```python
from build123d import *

# Parameters (mm, degrees)
SKETCH_1_R          = 50
EXTRUDE_1_DEPTH     = 15
SHELL_1_T           = -3
EXTRUDE_2_DEPTH     = 20
SKETCH_3_R          = 13
CUT_EXTRUDE_1_DEPTH = 79.89866919
SKETCH_4_R          = 16
SKETCH_4_R_2        = 13
EXTRUDE_3_DEPTH     = 12
SHELL_START         = 15
SHELL_5_DEPTH       = 20


# Read off the part's stored shape, not the designer's step: 薄殼5
with BuildPart() as part:
    # 草圖1 → 填料-伸長1 (new body)
    with BuildSketch(Plane.XY):
        Circle(SKETCH_1_R)
    extrude(amount=EXTRUDE_1_DEPTH)

    # 薄殼1
    shell_1_openings = [part.faces().sort_by_distance(p)[0] for p in [
        (0, 0, 0),
    ]]
    offset(amount=SHELL_1_T, openings=shell_1_openings, kind=Kind.INTERSECTION)

    # 草圖2 → 填料-伸長2 (add)
    with BuildSketch(Plane.XY.offset(15)):
        with BuildLine():
            Line((-15.588457268, 33), (-36.373066959, -3))
            ThreePointArc((-36.373066959, -3), (-36.373066959, -21), (-20.784609691, -30))
            Line((-20.784609691, -30), (20.784609691, -30))
            ThreePointArc((20.784609691, -30), (36.373066959, -21), (36.373066959, -3))
            Line((36.373066959, -3), (15.588457268, 33))
            ThreePointArc((15.588457268, 33), (0, 42), (-15.588457268, 33))
        make_face()
    extrude(amount=EXTRUDE_2_DEPTH)

    # 草圖3 → 除料-伸長1 (cut, through all)
    with BuildSketch(Plane.XY.offset(35)):
        with Locations((0, 24)):
            Circle(SKETCH_3_R)
        with Locations((-20.784609691, -12)):
            Circle(SKETCH_3_R)
        with Locations((20.784609691, -12)):
            Circle(SKETCH_3_R)
    extrude(amount=-CUT_EXTRUDE_1_DEPTH, mode=Mode.SUBTRACT)

    # 草圖4 → 填料-伸長3 (add)
    # profile 1 of 3: a face of its own
    with BuildSketch(Plane(origin=(0, 0, 12), x_dir=(-1, 0, 0), z_dir=(0, 0, -1))):
        with Locations(Location((0, 24, 0), (0, 0, 180))):
            Circle(SKETCH_4_R)
        with Locations(Location((0, 24, 0), (0, 0, 180))):
            Circle(SKETCH_4_R_2, mode=Mode.SUBTRACT)
    # profile 2 of 3: a face of its own
    with BuildSketch(Plane(origin=(0, 0, 12), x_dir=(-1, 0, 0), z_dir=(0, 0, -1))):
        with Locations(Location((20.784609691, -12, 0), (0, 0, 180))):
            Circle(SKETCH_4_R)
        with Locations(Location((20.784609691, -12, 0), (0, 0, 180))):
            Circle(SKETCH_4_R_2, mode=Mode.SUBTRACT)
    # profile 3 of 3: a face of its own
    with BuildSketch(Plane(origin=(0, 0, 12), x_dir=(-1, 0, 0), z_dir=(0, 0, -1))):
        with Locations(Location((-20.784609691, -12, 0), (0, 0, 180))):
            Circle(SKETCH_4_R)
        with Locations(Location((-20.784609691, -12, 0), (0, 0, 180))):
            Circle(SKETCH_4_R_2, mode=Mode.SUBTRACT)
    extrude(amount=EXTRUDE_3_DEPTH)

    # 薄殼5 outline → 薄殼5 (cut)
    with BuildSketch(Plane.XY.offset(SHELL_START)):
        with BuildLine():
            ThreePointArc((15.774263238, 26.67817462), (0, 8), (-15.774263238, 26.67817462))
            Line((-15.774263238, 26.67817462), (-30.991108566, 0.32182538))
            ThreePointArc((-30.991108566, 0.32182538), (-6.92820323, -4), (-15.216845328, -27))
            Line((-15.216845328, -27), (15.216845328, -27))
            ThreePointArc((15.216845328, -27), (6.92820323, -4), (30.991108566, 0.32182538))
            Line((30.991108566, 0.32182538), (15.774263238, 26.67817462))
        make_face()
    extrude(amount=SHELL_5_DEPTH, mode=Mode.SUBTRACT)


solid = part.part
```
Input: part model. Units: mm. Frame: model coordinates. A direction names the side the tool comes from. Round coordinates to 2 decimals unless told otherwise and drop trailing zeros. Order: outer loops, then holes, each group sorted by start corner. A loop starts at its lowest first (then second) coordinate and runs counter-clockwise, first axis right, second up. Notation, with made-up numbers: (-33.5, -1.5) - (1.5, -1.5) arc R13 ccw to (1.5, 6.5) - close; hole circle Ø5 at (1, -20). An arc over 180 degrees is marked (long way). One line per question, with ' | ' between items. Start each with the question number.
1) Cut plane D-D, the plane z = 31. Return the cut outline in (x, y), then the cut area to 3 significant figures.
2) Ray query, probe 1 along Y at (x, z) = (0, 7); probe 2 along Y at (x, z) = (0, 27.5); probe 3 along X at (y, z) = (35, 10.5). Return the intervals inside material, ascending.
3) Cut plane C-C, the plane y = 20. Return the cut outline in (x, z), then the cut area to 3 significant figures.
4) Pull-direction query (X, two-part tool) for faces 6 (the cylindrical face through (36.24, -21.23, 24.86)), 7 (the cylindrical face through (-7.127, -3.665, 24.86)), 8 (the cylindrical face through (0, 8, 25)), 9 (the flat face through (-9, -2, 35)); classes: +X half, -X half, draft (parallel to the pull), parting line (faces both ways), or undercut.
5) Set-up query: faces 1 (the flat face through (-1, -33, 15)), 2 (the cylindrical face through (33.184, -15.905, 17.745)), 3 (the flat face through (26.126, 14.748, 24.86)), 4 (the cylindrical face through (-36.503, -20.771, 24.86)), 5 (the flat face through (-1, 1, 12)). Return all of +Z, -Z, +X, -X, +Y, -Y with unobstructed straight access to the full face (end or side cutting, diameter ignored); none if empty.
6) Contact query for flat-ended pins moving along their axis: P1, Ø16, axis at x = 1.5, z = 24, coming from the +Y side; P2, Ø8, axis at x = -12, z = 4, coming from the -Y side; P3, Ø6, axis at y = 7, z = 19.5, coming from the +X side. Output: stop coordinate, or through.
7) Cut plane B-B, the plane x = 0. Return the cut outline in (y, z), then the cut area to 3 significant figures.
8) Cut plane A-A, the plane z = 4. Return the cut outline in (x, y).
Worked out:
1) outline: (-36.37, -3) arc R18 ccw to (-20.78, -30) - (20.78, -30) arc R18 ccw to (36.37, -3) - (15.59, 33) arc R18 ccw to (-15.59, 33) - close; hole circle Ø26 at (-20.78, -12); hole (-30.99, 0.32) arc R16 cw (long way) to (-15.22, -27) - (15.22, -27) arc R16 cw (long way) to (30.99, 0.32) - (15.77, 26.68) arc R16 cw (long way) to (-15.77, 26.68) - close; hole circle Ø26 at (0, 24); hole circle Ø26 at (20.78, -12) | area: 1,390 mm^2
2) probe 1: y = -50 to -47, 8 to 11, 37 to 40, 47 to 50 | probe 2: y = -30 to -27, 8 to 11, 37 to 42 | probe 3: x = -35.71 to -31.37, -11.62 to -6.93, 6.93 to 11.62, 31.37 to 35.71
3) outline: (-45.83, 0) - (-42.53, 0) - (-42.53, 12) - (-15.49, 12) - (-15.49, 0) - (-12.37, 0) - (-12.37, 35) - (-15.49, 35) - (-15.49, 15) - (-19.63, 15) - (-19.63, 35) - (-23.09, 35) - (-23.09, 15) - (-45.83, 15) - close; (12.37, 0) - (15.49, 0) - (15.49, 12) - (42.53, 12) - (42.53, 0) - (45.83, 0) - (45.83, 15) - (23.09, 15) - (23.09, 35) - (19.63, 35) - (19.63, 15) - (15.49, 15) - (15.49, 35) - (12.37, 35) - close | area: 618 mm^2
4) face 6: +X half | face 7: undercut | face 8: undercut | face 9: draft
5) face 1: +Z | face 2: +Z, -Z | face 3: +Z, +X, +Y | face 4: +Z, -X | face 5: -Z
6) P1: stops at y = 42 | P2: stops at y = -49.36 | P3: stops at x = 32.33
7) outline: (-50, 0) - (-47, 0) - (-47, 12) - (8, 12) - (8, 0) - (11, 0) - (11, 35) - (8, 35) - (8, 15) - (-27, 15) - (-27, 35) - (-30, 35) - (-30, 15) - (-50, 15) - close; (37, 0) - (40, 0) - (40, 12) - (47, 12) - (47, 0) - (50, 0) - (50, 15) - (42, 15) - (42, 35) - (37, 35) - close | area: 586 mm^2
8) outline: circle Ø100 at (0, 0); circle Ø32 at (-20.78, -12); circle Ø32 at (0, 24); circle Ø32 at (20.78, -12); hole circle Ø94 at (0, 0); hole circle Ø26 at (-20.78, -12); hole circle Ø26 at (0, 24); hole circle Ø26 at (20.78, -12)
